from build123d import *

# Parameters (mm, degrees)
F0_W     = 380
F0_H     = 380
F1_DEPTH = 350
F2_W     = 342
F2_H     = 312
F3_DEPTH = 342
F4_W     = 40
F4_H     = 40
F5_DEPTH = 150


with BuildPart() as f1:
    # F0 (on Top) → F1 (new body)
    with BuildSketch(Plane.XY):
        Rectangle(F0_W, F0_H)
    extrude(amount=F1_DEPTH)

    # F2 (on face) → F3 (cut)
    with BuildSketch(Plane.XZ.offset(190)):
        with Locations((0, 175)):
            Rectangle(F2_W, F2_H)
    extrude(amount=-F3_DEPTH, mode=Mode.SUBTRACT)

    # F4 (on face) → F5 (join)
    with BuildSketch(Plane(origin=(0, 0, 0), x_dir=(1, 0, 0), z_dir=(0, 0, -1))):
        with Locations((-170, 170)):
            Rectangle(F4_W, F4_H)
        with Locations((170, 170)):
            Rectangle(F4_W, F4_H)
        with Locations((170, -170)):
            Rectangle(F4_W, F4_H)
        with Locations((-170, -170)):
            Rectangle(F4_W, F4_H)
    extrude(amount=F5_DEPTH)


solid = f1.part
Design review of the part built by this model. Coordinates are the model's own, in mm. A direction names the side the tool comes from. Round coordinates to 2 decimals unless told otherwise and drop trailing zeros. Order: outer loops, then holes, each group sorted by start corner. A loop starts at its lowest first (then second) coordinate and runs counter-clockwise, first axis right, second up. Notation, with made-up numbers: M 61,61.5 L 117,61.5 A22 cw 117,83.5 Z; hole C 3,41 d8. An arc over 180 degrees is marked long. Answer as CSV lines item,"result". Start each with the question number.
1) Tool access review of faces 5 (the face through (-3, 190, 152)), 6 (the face through (150, -170, -74)), 7 (the face through (-171, -21, 173)), 8 (the face through (170, 150, -74)), 9 (the face through (190, -3, 152)): name each direction out of +Z, -Z, +X, -X, +Y, -Y from which nothing blocks a thin tool from reaching the whole face with its end or side.
2) The part is to be moulded in two halves that separate along Y. For faces 1 (the face through (-15, -190, 9)), 2 (the face through (-170, 150, -74)), 3 (the face through (-150, -170, -74)), 4 (the face through (-170, -150, -74)), say which applies: +Y half, -Y half, draft (parallel to the pull), parting line (faces both ways), or undercut.
3) Add section A-A (z = -55.5). Give the boundary of the cut face in (x, y).
4) Wall thickness on line 1 along X through (y, z) = (88, 104); line 2 along Z through (x, y) = (-72.5, -95); line 3 along Y through (x, z) = (152.5, -117): over which ranges is each line inside the solid? List them lowest first. Write a range as [from, to].
5) Add section C-C (x = -5). Give the boundary of the cut face in (y, z).
6) For pin 1 Ø3 at (x, z) = (-62, 180) entering from -Y; pin 2 Ø2 at (x, y) = (4.5, 85) entering from -Z, all flat-tipped, find the tip position at first contact; note any pin that passes through.
7) Add section B-B (y = -120). Give the boundary of the cut face in (x, z).
8) Add section D-D (z = 161). Give the boundary of the cut face in (x, y).
Resolved:
1,face 5,"+Z, -Z, +X, -X, +Y"
1,face 6,"-Z, +Y, -Y"
1,face 7,"-Y"
1,face 8,"-Z, +X, -X"
1,face 9,"+Z, -Z, +X, +Y, -Y"
2,face 1,"-Y half"
2,face 2,"undercut"
2,face 3,"draft"
2,face 4,"undercut"
3,outline,"M -190,-190 L -150,-190 L -150,-150 L -190,-150 Z; M -190,150 L -150,150 L -150,190 L -190,190 Z; M 150,-190 L 190,-190 L 190,-150 L 150,-150 Z; M 150,150 L 190,150 L 190,190 L 150,190 Z"
4,line 1,"[-190, -171], [171, 190]"
4,line 2,"[0, 19], [331, 350]"
4,line 3,"[-190, -150], [150, 190]"
5,outline,"M -190,0 L 190,0 L 190,350 L -190,350 L -190,331 L 152,331 L 152,19 L -190,19 Z"
6,pin 1,"y = 152"
6,pin 2,"z = 0"
7,outline,"M -190,0 L 190,0 L 190,350 L -190,350 Z; hole M -171,19 L 171,19 L 171,331 L -171,331 Z"
8,outline,"M -190,-190 L -171,-190 L -171,152 L 171,152 L 171,-190 L 190,-190 L 190,190 L -190,190 Z"
